For this review, take the finished solid that the model builds, in its own axes (mm). Coordinates: 2 decimals unless noted, no trailing zeros. Write each loop counter-clockwise with the first axis right and the second up, starting at its lowest first coordinate (ties: lowest second). Pieces come first, ordered by that corner, then holes.
1) Insertion check: P1, Ø0.6, axis at x = 2, z = -7, coming from the -Y side; P2, Ø0.6, axis at y = 0, z = -10, coming from the +X side (3 decimals); P3, Ø1.5, axis at x = -2, y = 1.5, coming from the -Z side. Each pin has a flat end and moves straight along its axis. Give the tip position at first contact, or say it passes through.
2) We need section A-A on z = -21.5. Write out the cut boundary in (x, y) (3 decimals).
3) To check wall thickness, follow line 1 along Y through (x, z) = (-2.05, -18); line 2 along Z through (x, y) = (-1.9, -2); line 3 along X through (y, z) = (-1.4, 4.5). State the ranges of each line that lie inside material, in increasing order.
4) Mouldability with a two-part tool opening along Y and no side actions: class faces 1 (the face through (0, 0, 0)), 2 (the face through (-0.54, -2.44, 3.61)) as pulls with the +Y half, pulls with the -Y half, needs draft (parallel to the pull), parting line crosses it, or undercut.
from build123d import *

# Parameters (mm, degrees)
F0_R     = 2.9
F1_DEPTH = 1
F2_R     = 2.5
F3_DEPTH = 8.7
F4_R     = 2.4
F5_W     = 0.5
F5_H     = 25
F5_H_2   = 26
F5_H_3   = 28
F5_H_4   = 27
F6_DEPTH = 0.25


with BuildPart() as f1:
    # F0 (on Top) → F1 (new body)
    with BuildSketch(Plane.XY):
        Circle(F0_R)
    extrude(amount=F1_DEPTH)

    # F2 (on Top) → F3 (join)
    with BuildSketch(Plane.XY):
        Circle(F2_R)
    extrude(amount=F3_DEPTH)

    # F4
    f4_edges = [f1.edges().sort_by_distance(p)[0] for p in [
        (-2.5, 0, 8.7),
    ]]
    fillet(f4_edges, radius=F4_R)

    # F5 (on Front) → F6 (join, symmetric)
    with BuildSketch(Plane.XZ):
        with Locations((-1.875, -12.5)):
            Rectangle(F5_W, F5_H)
        with Locations((-0.625, -13)):
            Rectangle(F5_W, F5_H_2)
        with Locations((0.625, -14)):
            Rectangle(F5_W, F5_H_3)
        with Locations((1.875, -13.5)):
            Rectangle(F5_W, F5_H_4)
    extrude(amount=F6_DEPTH, both=True)


solid = f1.part
Result:
1. P1: stops at y = -0.25
1. P2: stops at x = 2.125
1. P3: stops at z = 0
2. outline: (-2.125, -0.25) - (-1.625, -0.25) - (-1.625, 0.25) - (-2.125, 0.25) - close; (-0.875, -0.25) - (-0.375, -0.25) - (-0.375, 0.25) - (-0.875, 0.25) - close; (0.375, -0.25) - (0.875, -0.25) - (0.875, 0.25) - (0.375, 0.25) - close; (1.625, -0.25) - (2.125, -0.25) - (2.125, 0.25) - (1.625, 0.25) - close
3. line 1: y = -0.25 to 0.25
3. line 2: z = 0 to 1
3. line 3: x = -2.07 to 2.07
4. face 1: needs draft
4. face 2: parting line crosses it
